Geometry check sheet. Reference: drawing and pictorial views, mm from the part's lowest x, y, z. Give positions to 0.01 mm unless a question says otherwise; leave off trailing zeros. Loops run counter-clockwise (first coordinate to the right, second up) from the corner with the lowest first, then second, coordinate; pieces in that order, holes last. Notation, with made-up numbers: M -9.75,-14.5 L 10.25,-14.5 A17 cw 10.25,3.5 Z; hole C -3,-5 d5. An arc over 180 degrees is marked long. Use CSV: the item, a comma, the result in double quotes.
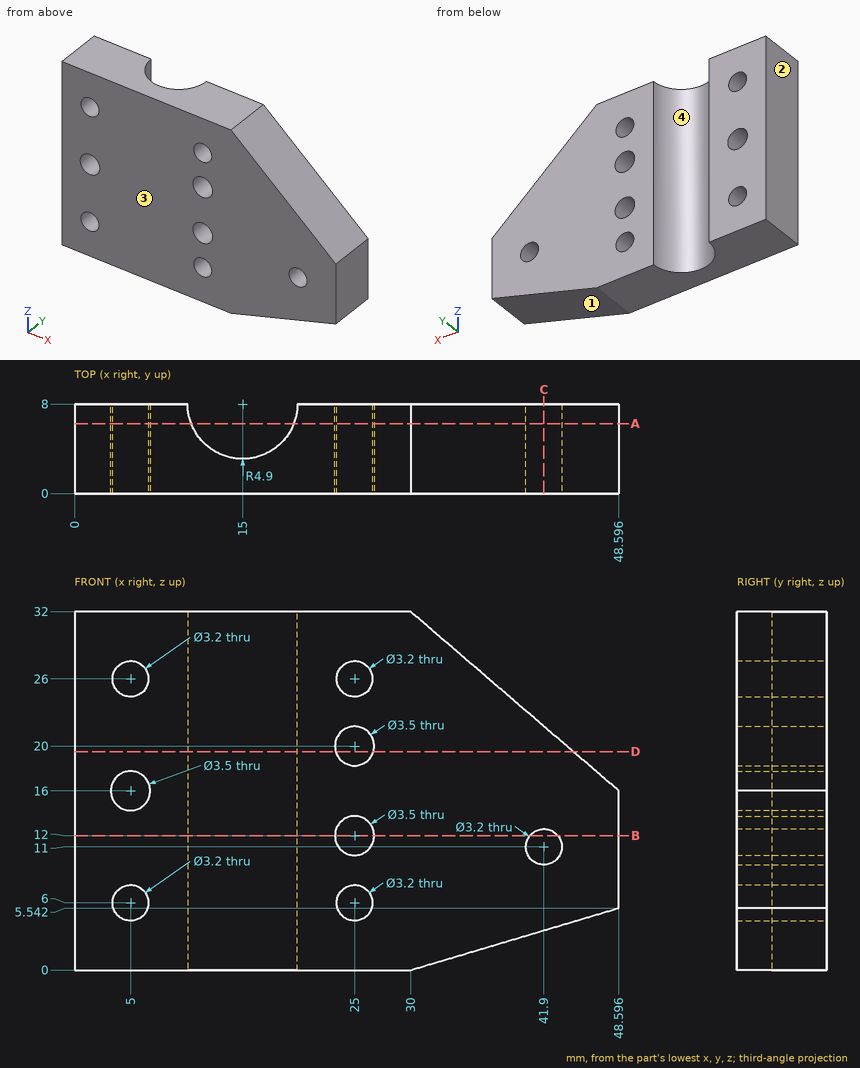
(1) Section check D-D on z = 19.5. Record the cut outline in (x, y).
Calculated:
outline,"M 0,0 L 23.32,0 L 23.32,8 L 19.9,8 A4.9 cw 10.1,8 L 0,8 Z; M 26.68,0 L 44.53,0 L 44.53,8 L 26.68,8 Z"
(2) Section check B-B on z = 12. Record the cut outline in (x, y), plus the area to 3 significant figures.
Calculated:
outline,"M 0,0 L 23.25,0 L 23.25,8 L 19.9,8 A4.9 cw 10.1,8 L 0,8 Z; M 26.75,0 L 40.65,0 L 40.65,8 L 26.75,8 Z; M 43.15,0 L 48.6,0 L 48.6,8 L 43.15,8 Z"
area,"303 mm²"
(3) Depth check by flat-ended pin: pin 1 Ø2.5 at (x, z) = (25, 6) entering from -Y. Enter the tip coordinate at first touch or a pass-through.
Calculated:
pin 1,"passes through"
(4) Section check A-A on y = 6.25. Count the separate pieces of the cut face and the enclosed holes in it, plus the area to 3 significant figures.
Calculated:
separate pieces,"2"
enclosed holes,"8"
area,"993 mm²"
(5) Section check C-C on x = 41.9. Record the cut outline in (y, z), plus the area to 3 significant figures.
Calculated:
outline,"M 0,3.55 L 8,3.55 L 8,9.4 L 0,9.4 Z; M 0,12.6 L 8,12.6 L 8,21.76 L 0,21.76 Z"
area,"120 mm²"
(6) Mould release check, pull along X, two halves, no side actions. Record for the marked faces 1, 2, 3 and 4: released by +X, released by -X, zero draft, split by the parting line, or undercut.
Calculated:
face 1,"released by +X"
face 2,"released by -X"
face 3,"zero draft"
face 4,"undercut"
(7) Scan lines: L1, parallel to Z at x = 25, y = 4.75; L2, parallel to X at y = 3.5, z = 11 (1 decimal); L3, parallel to X at y = 3.5, z = 17 (1 decimal). Record each from-to range of solid material in increasing order. Write a range as from..to.
Calculated:
L1,"z = 0..4.4, 7.6..10.25, 13.75..18.25, 21.75..24.4, 27.6..32"
L2,"x = 0..13.1, 16.9..23.6, 26.4..40.3, 43.5..48.6"
L3,"x = 0..3.6, 6.4..13.1, 16.9..47.4"
